Geometry: final body of the model. Coordinates: model frame, mm. Face numbers are marked on the shaded views. A direction names the side the tool comes from. Coordinates: 2 decimals unless noted, no trailing zeros. Write each loop counter-clockwise with the first axis right and the second up, starting at its lowest first coordinate (ties: lowest second). Pieces come first, ordered by that corner, then holes. Notation, with made-up numbers: (-19.5, -17) - (38.5, -17) arc R35 ccw to (38.5, 16) - close; hole circle Ø9 at (15, -34). An arc over 180 degrees is marked (long way). Answer as a JSON object with one key per item and string values. Group by question number.
Item 1: Section D-D on y = -17.5. Return loops of the section in (x, z), and give its area (3 significant figures).
Item 2: Set-up query: the marked faces 5 and 6. Return all of +Z, -Z, +X, -X, +Y, -Y with unobstructed straight access to the full face (end or side cutting, diameter ignored); none if empty.
Item 3: Section C-C on z = 1.75. Return loops of the section in (x, y).
Item 4: Line query: line 1 along Y through (x, z) = (-15.5, 5); line 2 along Y through (x, z) = (23.7, 5); line 3 along X through (y, z) = (16.5, 6). Output: solid intervals per line, ascending. Write a range as from..to.
Item 5: Mould query, pull axis X, two halves, no side actions, for the marked faces 1, 2, 3 and 4. Classes: pulls with the +X half, pulls with the -X half, needs draft (parallel to the pull), parting line crosses it, or undercut.
Item 6: Section A-A on z = 5. Return loops of the section in (x, y).
Item 7: First-contact query: pin 1 Ø3 at (x, y) = (-6.26, 3.28) entering from +Z; pin 2 Ø1.1 at (y, z) = (-11.5, 0.5) entering from -X. Flat tips, straight axial feed; report the tip coordinate or a pass-through.
Item 8: Section B-B on y = 11. Return loops of the section in (x, z), and give its area (3 significant figures).
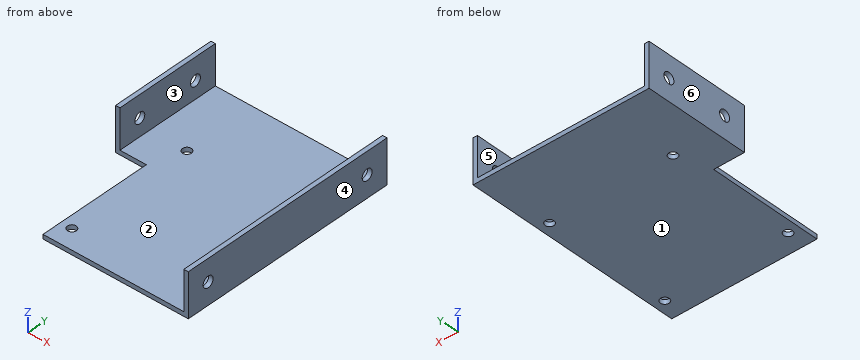
```python
from build123d import *

# Parameters (mm, degrees)
SKETCH1_W            = 40
SKETCH1_H            = 50
BOSS_EXTRUDE1_DEPTH  = 1
SKETCH2_W            = 5
SKETCH2_H            = 25
CUT_EXTRUDE1_DEPTH   = 1
SKETCH3_W            = 1
SKETCH3_H            = 25
BOSS_EXTRUDE2_DEPTH  = 10
SKETCH4_R            = 1.25
CUT_EXTRUDE3_DEPTH   = 63
SKETCH5_R            = 1.25
BOSS_EXTRUDE3_DEPTH  = 1
SKETCH6_W            = 40
SKETCH6_H            = 10
CUT_EXTRUDE4_DEPTH   = 9
SKETCH7_R            = 1.25
CUT_EXTRUDE5_DEPTH   = 53
SKETCH8_W            = 2
SKETCH8_H            = 25
CUT_EXTRUDE6_DEPTH   = 53
SKETCH9_W            = 7
SKETCH9_H            = 2
CUT_EXTRUDE8_DEPTH   = 53
SKETCH10_W           = 9
SKETCH10_H           = 20.650485051
BOSS_EXTRUDE4_DEPTH  = 1
SKETCH11_R           = 1.25
CUT_EXTRUDE9_DEPTH   = 1
SKETCH12_R           = 1.25
BOSS_EXTRUDE5_DEPTH  = 1
SKETCH13_R           = 1.25
BOSS_EXTRUDE6_DEPTH  = 1
SKETCH14_W           = 7
SKETCH14_H           = 1
BOSS_EXTRUDE7_DEPTH  = 1
SKETCH15_W           = 1
SKETCH15_H           = 9
BOSS_EXTRUDE8_DEPTH  = 9
SKETCH16_R           = 1.25
CUT_EXTRUDE10_DEPTH  = 9
SKETCH17_W           = 1
SKETCH17_H           = 31.406889679
BOSS_EXTRUDE9_DEPTH  = 9
SKETCH18_R           = 1.25
CUT_EXTRUDE11_DEPTH  = 9
SKETCH19_W           = 33
SKETCH19_H           = 1
BOSS_EXTRUDE10_DEPTH = 9
SKETCH20_R           = 1.25
CUT_EXTRUDE12_DEPTH  = 9
SKETCH21_R           = 1
CUT_EXTRUDE13_DEPTH  = 10
SKETCH22_W           = 33
SKETCH22_H           = 1
CUT_EXTRUDE14_DEPTH  = 9
SKETCH23_W           = 1
SKETCH23_H           = 1
BOSS_EXTRUDE11_DEPTH = 9


with BuildPart() as part:
    # Sketch1 → Boss-Extrude1 (new body)
    with BuildSketch(Plane.XY):
        with Locations((4.242424242, -5.173160173)):
            Rectangle(SKETCH1_W, SKETCH1_H)
    extrude(amount=BOSS_EXTRUDE1_DEPTH)

    # Sketch2 → Cut-Extrude1 (cut)
    with BuildSketch(Plane.XY.offset(1)):
        with Locations((-13.257575758, -17.673160173)):
            Rectangle(SKETCH2_W, SKETCH2_H)
    extrude(amount=-CUT_EXTRUDE1_DEPTH, mode=Mode.SUBTRACT)

    # Sketch3 → Boss-Extrude2 (add)
    with BuildSketch(Plane(origin=(0, 0, 0), x_dir=(-1, 0, 0), z_dir=(0, 0, -1))):
        with Locations((15.257575758, 7.326839827)):
            Rectangle(SKETCH3_W, SKETCH3_H)
        with Locations((-23.742424242, 7.326839827)):
            Rectangle(SKETCH3_W, SKETCH3_H)
    extrude(amount=-BOSS_EXTRUDE2_DEPTH)

    # Sketch4 → Cut-Extrude3 (cut)
    with BuildSketch(Plane(origin=(24.242424242, 0, 0), x_dir=(0, 0, -1), z_dir=(1, 0, 0))):
        with Locations((-5, -0.173160173)):
            Circle(SKETCH4_R)
        with Locations((-5, 14.826839827)):
            Circle(SKETCH4_R)
    extrude(amount=-CUT_EXTRUDE3_DEPTH, mode=Mode.SUBTRACT)

    # Sketch5 → Boss-Extrude3 (add)
    with BuildSketch(Plane(origin=(24.242424242, 0, 0), x_dir=(0, 0, -1), z_dir=(1, 0, 0))):
        with Locations((-5, -0.173160173)):
            Circle(SKETCH5_R)
    extrude(amount=-BOSS_EXTRUDE3_DEPTH)

    # Sketch6 → Cut-Extrude4 (cut)
    with BuildSketch(Plane.XY.offset(10)):
        with Locations((4.242424242, -0.173160173)):
            Rectangle(SKETCH6_W, SKETCH6_H)
    extrude(amount=-CUT_EXTRUDE4_DEPTH, mode=Mode.SUBTRACT)

    # Sketch7 → Cut-Extrude5 (cut)
    with BuildSketch(Plane.ZY.offset(15.757575758)):
        with Locations((5, 9.826839827)):
            Circle(SKETCH7_R)
    extrude(amount=-CUT_EXTRUDE5_DEPTH, mode=Mode.SUBTRACT)

    # Sketch8 → Cut-Extrude6 (cut)
    with BuildSketch(Plane.XY.offset(1)):
        with Locations((-9.757575758, -17.673160173)):
            Rectangle(SKETCH8_W, SKETCH8_H)
    extrude(amount=-CUT_EXTRUDE6_DEPTH, mode=Mode.SUBTRACT)

    # Sketch9 → Cut-Extrude8 (cut)
    with BuildSketch(Plane.XY.offset(1)):
        with Locations((-12.257575758, -4.173160173)):
            Rectangle(SKETCH9_W, SKETCH9_H)
    extrude(amount=-CUT_EXTRUDE8_DEPTH, mode=Mode.SUBTRACT)

    # Sketch10 → Boss-Extrude4 (add)
    with BuildSketch(Plane(origin=(24.242424242, 0, 0), x_dir=(0, 0, -1), z_dir=(1, 0, 0))):
        with Locations((-5.5, -5.498402699)):
            Rectangle(SKETCH10_W, SKETCH10_H)
    extrude(amount=-BOSS_EXTRUDE4_DEPTH)

    # Sketch11 → Cut-Extrude9 (cut)
    with BuildSketch(Plane(origin=(24.242424242, 0, 0), x_dir=(0, 0, -1), z_dir=(1, 0, 0))):
        with Locations((-5, -10.823645224)):
            Circle(SKETCH11_R)
    extrude(amount=-CUT_EXTRUDE9_DEPTH, mode=Mode.SUBTRACT)

    # Sketch12 → Boss-Extrude5 (add)
    with BuildSketch(Plane(origin=(24.242424242, 0, 0), x_dir=(0, 0, -1), z_dir=(1, 0, 0))):
        with Locations((-5, 9.826839827)):
            Circle(SKETCH12_R)
    extrude(amount=-BOSS_EXTRUDE5_DEPTH)

    # Sketch13 → Boss-Extrude6 (add)
    with BuildSketch(Plane.ZY.offset(15.757575758)):
        with Locations((5, 9.826839827)):
            Circle(SKETCH13_R)
    extrude(amount=-BOSS_EXTRUDE6_DEPTH)

    # Sketch14 → Boss-Extrude7 (add)
    with BuildSketch(Plane.XY.offset(1)):
        with Locations((-12.257575758, -3.673160173)):
            Rectangle(SKETCH14_W, SKETCH14_H)
    extrude(amount=-BOSS_EXTRUDE7_DEPTH)

    # Sketch15 → Boss-Extrude8 (add)
    with BuildSketch(Plane.XY.offset(1)):
        with Locations((-15.257575758, 0.326839827)):
            Rectangle(SKETCH15_W, SKETCH15_H)
    extrude(amount=BOSS_EXTRUDE8_DEPTH)

    # Sketch16 → Cut-Extrude10 (cut)
    with BuildSketch(Plane.ZY.offset(15.757575758)):
        with Locations((5, 14.826839827)):
            Circle(SKETCH16_R)
        with Locations((5, 0.826839827)):
            Circle(SKETCH16_R)
    extrude(amount=-CUT_EXTRUDE10_DEPTH, mode=Mode.SUBTRACT)

    # Sketch17 → Boss-Extrude9 (add)
    with BuildSketch(Plane.XY.offset(1)):
        with Locations((23.742424242, -14.469715334)):
            Rectangle(SKETCH17_W, SKETCH17_H)
    extrude(amount=BOSS_EXTRUDE9_DEPTH)

    # Sketch18 → Cut-Extrude11 (cut)
    with BuildSketch(Plane(origin=(24.242424242, 0, 0), x_dir=(0, 0, -1), z_dir=(1, 0, 0))):
        with Locations((-5, -25.173160173)):
            Circle(SKETCH18_R)
    extrude(amount=-CUT_EXTRUDE11_DEPTH, mode=Mode.SUBTRACT)

    # Sketch19 → Boss-Extrude10 (add)
    with BuildSketch(Plane.XY.offset(1)):
        with Locations((7.742424242, -29.673160173)):
            Rectangle(SKETCH19_W, SKETCH19_H)
    extrude(amount=BOSS_EXTRUDE10_DEPTH)

    # Sketch20 → Cut-Extrude12 (cut)
    with BuildSketch(Plane.XZ.offset(30.173160173)):
        with Locations((-3.757575758, 5)):
            Circle(SKETCH20_R)
        with Locations((19.242424242, 5)):
            Circle(SKETCH20_R)
    extrude(amount=-CUT_EXTRUDE12_DEPTH, mode=Mode.SUBTRACT)

    # Sketch21 → Cut-Extrude13 (cut)
    with BuildSketch(Plane(origin=(0, 0, 0), x_dir=(-1, 0, 0), z_dir=(0, 0, -1))):
        with Locations((-21.742424242, 3.326839827)):
            Circle(SKETCH21_R)
        with Locations((6.257575758, 3.27845273)):
            Circle(SKETCH21_R)
        with Locations((6.257575758, -25.673160173)):
            Circle(SKETCH21_R)
        with Locations((-21.742424242, -25.673160173)):
            Circle(SKETCH21_R)
    extrude(amount=-CUT_EXTRUDE13_DEPTH, mode=Mode.SUBTRACT)

    # Sketch22 → Cut-Extrude14 (cut)
    with BuildSketch(Plane.XY.offset(10)):
        with Locations((7.742424242, -29.673160173)):
            Rectangle(SKETCH22_W, SKETCH22_H)
    extrude(amount=-CUT_EXTRUDE14_DEPTH, mode=Mode.SUBTRACT)

    # Sketch23 → Boss-Extrude11 (add)
    with BuildSketch(Plane.XY.offset(1)):
        with Locations((23.742424242, -29.673160173)):
            Rectangle(SKETCH23_W, SKETCH23_H)
    extrude(amount=BOSS_EXTRUDE11_DEPTH)


solid = part.part
```
Checks:
{
 "1": {"outline": "(-8.76, 0) - (24.24, 0) - (24.24, 10) - (23.24, 10) - (23.24, 1) - (-8.76, 1) - close", "area": "42.0 mm^2"},
 "2": {"face 5": "+Z, +Y, -Y", "face 6": "+Z, -Z, -X, +Y, -Y"},
 "3": {"outline": "(-15.76, -4.17) - (-14.76, -4.17) - (-14.76, 19.83) - (-15.76, 19.83) - close; (23.24, -30.17) - (24.24, -30.17) - (24.24, 19.83) - (23.24, 19.83) - close"},
 "4": {"line 1": "-4.17..-0.42, 2.08..13.58, 16.08..19.83", "line 2": "-30.17..-26.42, -23.92..13.58, 16.08..19.83", "line 3": "-15.76..-14.76, 23.24..24.24"},
 "5": {"face 1": "needs draft", "face 2": "undercut", "face 3": "undercut", "face 4": "pulls with the +X half"},
 "6": {"outline": "(-15.76, -4.17) - (-14.76, -4.17) - (-14.76, -0.42) - (-15.76, -0.42) - close; (-15.76, 2.08) - (-14.76, 2.08) - (-14.76, 13.58) - (-15.76, 13.58) - close; (-15.76, 16.08) - (-14.76, 16.08) - (-14.76, 19.83) - (-15.76, 19.83) - close; (23.24, -30.17) - (24.24, -30.17) - (24.24, -26.42) - (23.24, -26.42) - close; (23.24, -23.92) - (24.24, -23.92) - (24.24, 13.58) - (23.24, 13.58) - close; (23.24, 16.08) - (24.24, 16.08) - (24.24, 19.83) - (23.24, 19.83) - close"},
 "7": {"pin 1": "z = 1", "pin 2": "x = -8.76"},
 "8": {"outline": "(-15.76, 0) - (24.24, 0) - (24.24, 10) - (23.24, 10) - (23.24, 1) - (-14.76, 1) - (-14.76, 10) - (-15.76, 10) - close", "area": "58.0 mm^2"}
}
